The listing builds one solid part. Answer for the finished solid, in the listing's coordinates (mm). A direction names the side the tool comes from. Coordinates: 2 decimals unless noted, no trailing zeros. One line per question, with ' | ' between items.
from build123d import *

# Parameters (mm, degrees)
BOSS_EXTRUDE1_DEPTH = 80
SKETCH2_R           = 1.75
CUT_EXTRUDE1_DEPTH  = 87.654486324
SKETCH3_R           = 4.75
CUT_EXTRUDE2_DEPTH  = 3
SKETCH4_R           = 1.75
CUT_EXTRUDE3_DEPTH  = 89.36854644
LPATTERN1_COUNT     = 8
LPATTERN1_PITCH     = 10


with BuildPart() as part:
    # Sketch1 → Boss-Extrude1 (new body)
    with BuildSketch(Plane.XY):
        Polygon((16, 14), (25, 14), (25, -14), (-25, -14), (-25, 14), (-16, 14), (-16, -8), (16, -8), align=None)
    extrude(amount=BOSS_EXTRUDE1_DEPTH)

    # Sketch2 → Cut-Extrude1 (cut, through all)
    with BuildSketch(Plane(origin=(0, -8, 0), x_dir=(1, 0, 0), z_dir=(0, 1, 0))):
        with Locations(Location((-10, -5, 0), (0, 0, 180))):
            Circle(SKETCH2_R)
        with Locations(Location((10, -5, 0), (0, 0, 180))):
            Circle(SKETCH2_R)
    cut_extrude1 = extrude(amount=-CUT_EXTRUDE1_DEPTH, mode=Mode.SUBTRACT)

    # Sketch3 → Cut-Extrude2 (cut)
    with BuildSketch(Plane(origin=(0, -8, 0), x_dir=(1, 0, 0), z_dir=(0, 1, 0))):
        with Locations(Location((-10, -5, 0), (0, 0, 180))):
            Circle(SKETCH3_R)
        with Locations(Location((10, -5, 0), (0, 0, 180))):
            Circle(SKETCH3_R)
    cut_extrude2 = extrude(amount=-CUT_EXTRUDE2_DEPTH, mode=Mode.SUBTRACT)

    # Sketch4 → Cut-Extrude3 (cut, through all)
    with BuildSketch(Plane(origin=(0, 14, 0), x_dir=(1, 0, 0), z_dir=(0, 1, 0))):
        with Locations(Location((-20.5, -5, 0), (0, 0, 180))):
            Circle(SKETCH4_R)
        with Locations(Location((20.5, -5, 0), (0, 0, 180))):
            Circle(SKETCH4_R)
    cut_extrude3 = extrude(amount=-CUT_EXTRUDE3_DEPTH, mode=Mode.SUBTRACT)

    # LPattern1: Cut-Extrude1, Cut-Extrude2, Cut-Extrude3 ×8
    with Locations(*[(0, 0, i * LPATTERN1_PITCH) for i in range(1, LPATTERN1_COUNT)]):
        add(cut_extrude1, mode=Mode.SUBTRACT)
        add(cut_extrude2, mode=Mode.SUBTRACT)
        add(cut_extrude3, mode=Mode.SUBTRACT)


solid = part.part
Item 1: Find the intervals of material crossed by line 1 (X direction, y = 7.25, z = 65); line 2 (X direction, y = 0.25, z = 19); line 3 (Y direction, x = -7.5, z = 4), in increasing order. Write a range as [from, to].
Taken from the geometry:
line 1: x = [-25, -22.25], [-18.75, -16], [16, 18.75], [22.25, 25] | line 2: x = [-25, -16], [16, 25] | line 3: y = [-14, -11]
Item 2: Each of these flat-tipped pins is pushed along its axis until it touches: pin 1 Ø3 at (x, z) = (-10, 55) entering from -Y; pin 2 Ø10.5 at (x, z) = (10.5, 15.5) entering from +Y; pin 3 Ø3 at (x, z) = (9.5, 33.5) entering from +Y. Where does it stop, or does it pass through?
Taken from the geometry:
pin 1: passes through | pin 2: stops at y = -8 | pin 3: stops at y = -11
Item 3: Find section A-A, the plane y = 8.5. State how many separate pieces and enclosed holes the cut face has, plus the area to 3 significant figures.
Taken from the geometry:
separate pieces: 2 | enclosed holes: 16 | area: 1,290 mm2
Item 4: The mould has two halves that part along X. Classify faces 1 (the face through (10.62, -9.48, 19.71)), 2 (the face through (25, 0, 39)): pulls with the +X half, pulls with the -X half, needs draft (parallel to the pull), parting line crosses it, or undercut.
Taken from the geometry:
face 1: undercut | face 2: pulls with the +X half
Item 5: Which of the six approach directions +Z, -Z, +X, -X, +Y, -Y give full straight-line access (tool end or side, diameter ignored) to faces 3 (the face through (0, -8, 39)), 4 (the face through (8, -11, 75)), 5 (the face through (21.89, 0.2, 53.94))?
Taken from the geometry:
face 3: +Z, -Z, +Y | face 4: +Y | face 5: +Y, -Y
